Can you work these out from the model? Positions are in its coordinate system, mm. A direction names the side the tool comes from. Give positions to 0.01 mm unless a question says otherwise; leave off trailing zeros. Loops run counter-clockwise (first coordinate to the right, second up) from the corner with the lowest first, then second, coordinate; pieces in that order, holes last. Notation, with made-up numbers: M -37.5,4.5 L -26.5,4.5 A23 ccw -26.5,16.5 Z; hole C -9.75,52 d6. An arc over 180 degrees is marked long. Answer as a JSON object with one key per item and string values.
```python
from build123d import *

# Parameters (mm, degrees)
SKETCH23_W            = 55.7
SKETCH23_H            = 37.7
SKETCH23_W_2          = 47.7
SKETCH23_H_2          = 29.7
BOSS_EXTRUDE11_DEPTH  = 34.1
BOSS_EXTRUDE3_DEPTH   = 6
BOSS_EXTRUDE3_2_DEPTH = 6
SKETCH19_W            = 6
SKETCH19_H            = 20
SKETCH19_W_2          = 20
SKETCH19_H_2          = 6
SKETCH19_W_3          = 8
SKETCH19_H_3          = 45.451128654
SKETCH19_W_4          = 23.872388302
SKETCH19_H_4          = 8
BOSS_EXTRUDE10_DEPTH  = 16
FILLET6_R             = 16
FILLET7_R             = 2
SKETCH11_R            = 1.2
CUT_EXTRUDE1_DEPTH    = 121.03618278
SKETCH21_R            = 2.35
CUT_EXTRUDE2_DEPTH    = 2.4
CUT_EXTRUDE3_START    = -2.4
SKETCH22_R            = 2.35
CUT_EXTRUDE3_DEPTH    = 2.4


with BuildPart() as part:
    # Sketch23 → Boss-Extrude11 (new body)
    with BuildSketch(Plane(origin=(0, 0, 0), x_dir=(1, 0, 0), z_dir=(0, 1, 0))):
        with Locations((27.85, -18.85)):
            Rectangle(SKETCH23_W, SKETCH23_H)
        with Locations((27.85, -18.85)):
            Rectangle(SKETCH23_W_2, SKETCH23_H_2, mode=Mode.SUBTRACT)
    extrude(amount=-BOSS_EXTRUDE11_DEPTH)



with BuildPart() as body_2:
    # Sketch12 → Boss-Extrude3 (new body)
    with BuildSketch(Plane(origin=(0, 0, 0), x_dir=(1, 0, 0), z_dir=(0, 1, 0))):
        Polygon((0, -83.151128654), (-12.2428, -83.151128654), (-18.2428, -83.151128654), (-18.2428, -63.151128654), (-12.2428, -63.151128654), (0, -63.151128654), (8, -63.151128654), (8, -83.151128654), align=None)
    extrude(amount=BOSS_EXTRUDE3_DEPTH)


with BuildPart() as body_3:
    # Sketch12 → Boss-Extrude3 2 (new body)
    with BuildSketch(Plane(origin=(0, 0, 0), x_dir=(1, 0, 0), z_dir=(0, 1, 0))):
        Polygon((59.572388302, -8), (59.572388302, 0), (59.572388302, 12.2428), (59.572388302, 18.2428), (79.572388302, 18.2428), (79.572388302, 12.2428), (79.572388302, 0), (79.572388302, -8), align=None)
    extrude(amount=BOSS_EXTRUDE3_2_DEPTH)


with BuildPart() as part_1:
    add(part.part)

    add(body_2.part)  # Boss-Extrude10 merges body 2

    add(body_3.part)  # Boss-Extrude10 merges body 3
    # Sketch19 → Boss-Extrude10 (add)
    with BuildSketch(Plane(origin=(0, 0, 0), x_dir=(1, 0, 0), z_dir=(0, 1, 0))):
        with Locations((-15.2428, -73.151128654)):
            Rectangle(SKETCH19_W, SKETCH19_H)
        with Locations((69.572388302, 15.2428)):
            Rectangle(SKETCH19_W_2, SKETCH19_H_2)
        with Locations((4, -60.425564327)):
            Rectangle(SKETCH19_W_3, SKETCH19_H_3)
        with Locations((67.636194151, -4)):
            Rectangle(SKETCH19_W_4, SKETCH19_H_4)
    extrude(amount=-BOSS_EXTRUDE10_DEPTH)

    # Fillet6
    fillet6_edges = [part_1.edges().sort_by_distance(p)[0] for p in [
        (79.572388302, -16, 4),
        (4, -16, 83.151128654),
    ]]
    fillet(fillet6_edges, radius=FILLET6_R)

    # Fillet7
    fillet7_edges = [part_1.edges().sort_by_distance(p)[0] for p in [
        (74.886096801, -11.313708499, 8),
        (8, 3, 83.151128654),
        (8, -16, 52.425564327),
        (8, -11.313708499, 78.464837153),
        (55.7, -34.1, 18.85),
        (4, 0, 63.151128654),
        (-18.2428, -5, 63.151128654),
        (-18.2428, -5, 83.151128654),
        (8, 6, 73.151128654),
        (-5.1214, 6, 63.151128654),
        (-18.2428, 6, 73.151128654),
        (-5.1214, 6, 83.151128654),
        (59.636194151, -16, 8),
        (79.572388302, -5, -18.2428),
        (59.572388302, 0, 4),
        (59.572388302, -5, -18.2428),
        (69.572388302, 6, 8),
        (79.572388302, 6, -5.1214),
        (69.572388302, 6, -18.2428),
        (59.572388302, 6, -5.1214),
        (-18.2428, -16, 73.151128654),
        (-12.2428, -16, 73.151128654),
        (55.7, -17.05, 37.7),
        (69.572388302, -16, -18.2428),
        (69.572388302, -16, -12.2428),
        (27.85, -34.1, 37.7),
        (79.572388302, 3, 8),
    ]]
    fillet(fillet7_edges, radius=FILLET7_R)

    # Sketch11 → Cut-Extrude1 (cut, through all)
    with BuildSketch(Plane(origin=(0, 0, 0), x_dir=(-1, 0, 0), z_dir=(0, 0, -1))):
        with Locations(Location((-19.011079079, -11, 0), (0, 0, 180))):
            Circle(SKETCH11_R)
        with Locations(Location((-19.011079079, -23, 0), (0, 0, 180))):
            Circle(SKETCH11_R)
        with Locations(Location((-43.01107908, -11, 0), (0, 0, 180))):
            Circle(SKETCH11_R)
        with Locations(Location((-43.011079079, -23, 0), (0, 0, 180))):
            Circle(SKETCH11_R)
    extrude(amount=-CUT_EXTRUDE1_DEPTH, mode=Mode.SUBTRACT)

    # Sketch21 → Cut-Extrude2 (cut)
    with BuildSketch(Plane.XY.offset(37.7)):
        with Locations((19.011079079, -11)):
            Circle(SKETCH21_R)
        with Locations((43.01107908, -11)):
            Circle(SKETCH21_R)
        with Locations((19.011079079, -23)):
            Circle(SKETCH21_R)
        with Locations((43.011079079, -23)):
            Circle(SKETCH21_R)
    extrude(amount=-CUT_EXTRUDE2_DEPTH, mode=Mode.SUBTRACT)

    # Sketch22 → Cut-Extrude3 (cut)
    with BuildSketch(Plane(origin=(0, 0, 0), x_dir=(-1, 0, 0), z_dir=(0, 0, -1)).offset(CUT_EXTRUDE3_START)):
        with Locations(Location((-43.01107908, -11, 0), (0, 0, 180))):
            Circle(SKETCH22_R)
        with Locations(Location((-43.011079079, -23, 0), (0, 0, 180))):
            Circle(SKETCH22_R)
        with Locations(Location((-19.011079079, -11, 0), (0, 0, 180))):
            Circle(SKETCH22_R)
        with Locations(Location((-19.011079079, -23, 0), (0, 0, 180))):
            Circle(SKETCH22_R)
    extrude(amount=CUT_EXTRUDE3_DEPTH, mode=Mode.SUBTRACT)


solid = part_1.part
```
1) Suppose I cut it at A-A, the plane z = 31. Write out the boundary of the cut face in (x, y), and give its area (3 significant figures).
Answer list:
{"outline": "M 0,-34.1 L 4,-34.1 L 4,0 L 0,0 Z; M 51.7,-34.1 L 53.7,-34.1 A2 ccw 55.7,-32.1 L 55.7,0 L 51.7,0 Z", "area": "272 mm^2"}
2) Will these pins go through, and if not, where does the flat tip stop? pin 1 Ø5 at (x, y) = (20, -23.5) entering from +Z; pin 2 Ø4 at (x, y) = (19.01, -11) entering from +Z; pin 3 Ø12 at (x, z) = (32, 2.5) entering from +Y; pin 4 Ø1.4 at (x, y) = (43.01, -23) entering from -Z.
Answer list:
{"pin 1": "z = 37.7", "pin 2": "z = 35.3", "pin 3": "y = 0", "pin 4": "through"}
3) For faces 1 (the flat face through (3, -16, 52)), 2 (the cylindrical face through (3.042, -11.437, 78.34)), 3 (the flat face through (28, -17, 33.7)), 4 (the flat face through (-12.243, -7, 73)), 5 (the flat face through (42, -24, 2.4)), which set-ups out of +Z, -Z, +X, -X, +Y, -Y let a thin tool reach every point of the face, with its end or its side?
Answer list:
{"face 1": "+Z, +X, -X, -Y", "face 2": "+Z, +X, -Y", "face 3": "+Y, -Y", "face 4": "+Z, -Z, -Y", "face 5": "-Z"}
4) Suppose I cut it at D-D, the plane z = 52. Write out the boundary of the cut face in (x, y), and give its area (3 significant figures).
Answer list:
{"outline": "M 0,-16 L 6,-16 A2 ccw 8,-14 L 8,0 L 0,0 Z", "area": "127 mm^2"}
5) Suppose I cut it at B-B, the plane y = -29.5. Write out the boundary of the cut face in (x, z), and give its area (3 significant figures).
Answer list:
{"outline": "M 0,0 L 55.7,0 L 55.7,35.7 A2 ccw 53.7,37.7 L 0,37.7 Z; hole M 4,4 L 51.7,4 L 51.7,33.7 L 4,33.7 Z", "area": "682 mm^2"}
6) If we mould it in two halves opening along X, with no side actions, what happens to faces 6 (the cylindrical face through (18.06, -10.27, 34.49)), 7 (the flat face through (69, -5, -18.243))? For each: +X half, -X half, draft (parallel to the pull), parting line (faces both ways), or undercut.
Answer list:
{"face 6": "undercut", "face 7": "draft"}
7) Suppose I cut it at C-C, the plane y = -23. Give the number of separate pieces and of enclosed holes in the cut face, and give its area (3 significant figures).
Answer list:
{"separate pieces": "4", "enclosed holes": "0", "area": "622 mm^2"}
8) Please list where these lines run through material, in increasing order: line 1 along X through (y, z) = (-23, 3); line 2 along Z through (x, y) = (17, -32); line 3 along X through (y, z) = (-11, 3.1). Write a range as from..to.
Answer list:
{"line 1": "0..17.81, 20.21..41.81, 44.21..55.7", "line 2": "0..4, 33.7..37.7", "line 3": "0..17.81, 20.21..41.81, 44.21..75.19"}
